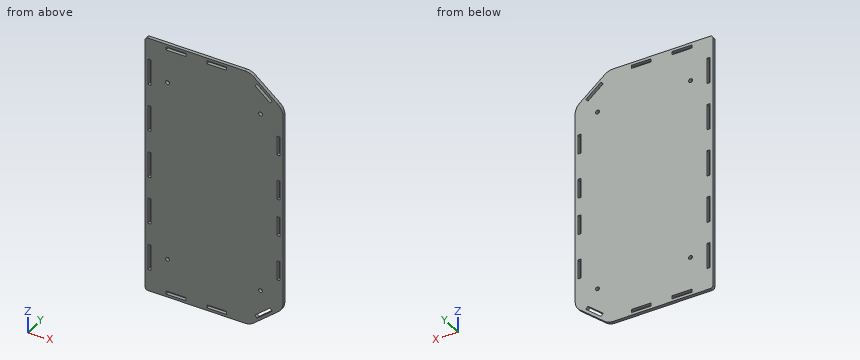
from build123d import *

# Parameters (mm, degrees)
SKETCH1_R           = 1.5
SKETCH1_W           = 15
SKETCH1_H           = 2.5
SKETCH1_W_2         = 2.5
SKETCH1_H_2         = 15
SKETCH1_H_3         = 20
BOSS_EXTRUDE1_DEPTH = 1.25
FILLET1_R           = 10
FILLET2_R           = 2


with BuildPart() as part:
    # Sketch1 → Boss-Extrude1 (new, symmetric)
    with BuildSketch(Plane(origin=(0, 0, 0), x_dir=(1, 0, 0), z_dir=(0, 1, 0))):
        Polygon((-52, -100), (27, -100), (52, -79.022509221), (52, 79.022509221), (27, 100), (-52, 100), align=None)
        with Locations(Location((35.127158073, -70, 0), (0, 0, 270))):
            Circle(SKETCH1_R, mode=Mode.SUBTRACT)
        with Locations(Location((35.127158073, 70, 0), (0, 0, 270))):
            Circle(SKETCH1_R, mode=Mode.SUBTRACT)
        with Locations(Location((-35.127158073, 70, 0), (0, 0, 270))):
            Circle(SKETCH1_R, mode=Mode.SUBTRACT)
        with Locations(Location((-35.127158073, -70, 0), (0, 0, 270))):
            Circle(SKETCH1_R, mode=Mode.SUBTRACT)
        with Locations((-28.71, -96.75)):
            Rectangle(SKETCH1_W, SKETCH1_H, mode=Mode.SUBTRACT)
        with Locations((2.08, -96.75)):
            Rectangle(SKETCH1_W, SKETCH1_H, mode=Mode.SUBTRACT)
        with Locations((-28.71, 96.75)):
            Rectangle(SKETCH1_W, SKETCH1_H, mode=Mode.SUBTRACT)
        with Locations((2.08, 96.75)):
            Rectangle(SKETCH1_W, SKETCH1_H, mode=Mode.SUBTRACT)
        Polygon((30.862122433, -90.884961689), (32.469091457, -92.800072797), (43.959758104, -83.158258651), (42.35278908, -81.243147544), align=None, mode=Mode.SUBTRACT)
        with Locations((48.75, 14.424124759)):
            Rectangle(SKETCH1_W_2, SKETCH1_H_2, mode=Mode.SUBTRACT)
        with Locations((48.75, -49.424124759)):
            Rectangle(SKETCH1_W_2, SKETCH1_H_2, mode=Mode.SUBTRACT)
        with Locations((48.75, -14.424124759)):
            Rectangle(SKETCH1_W_2, SKETCH1_H_2, mode=Mode.SUBTRACT)
        with Locations((48.75, 49.424124759)):
            Rectangle(SKETCH1_W_2, SKETCH1_H_2, mode=Mode.SUBTRACT)
        Polygon((42.35278908, 81.243147544), (30.862122433, 90.884961689), (32.469091457, 92.800072797), (43.959758104, 83.158258651), align=None, mode=Mode.SUBTRACT)
        with Locations((-48.75, -36.666666667)):
            Rectangle(SKETCH1_W_2, SKETCH1_H_3, mode=Mode.SUBTRACT)
        with Locations((-48.75, -73.333333333)):
            Rectangle(SKETCH1_W_2, SKETCH1_H_3, mode=Mode.SUBTRACT)
        with Locations((-48.75, 0)):
            Rectangle(SKETCH1_W_2, SKETCH1_H_3, mode=Mode.SUBTRACT)
        with Locations((-48.75, 36.666666667)):
            Rectangle(SKETCH1_W_2, SKETCH1_H_3, mode=Mode.SUBTRACT)
        with Locations((-48.75, 73.333333333)):
            Rectangle(SKETCH1_W_2, SKETCH1_H_3, mode=Mode.SUBTRACT)
    extrude(amount=BOSS_EXTRUDE1_DEPTH, both=True)

    # Fillet1
    fillet1_edges = [part.edges().sort_by_distance(p)[0] for p in [
        (27, 0, -100),
        (52, 0, -79.022509221),
        (52, 0, 79.022509221),
        (27, 0, 100),
    ]]
    fillet(fillet1_edges, radius=FILLET1_R)

    # Fillet2
    fillet2_edges = [part.edges().sort_by_distance(p)[0] for p in [
        (-52, 0, 100),
        (-52, 0, -100),
    ]]
    fillet(fillet2_edges, radius=FILLET2_R)


solid = part.part
Work out the finished part from the listing and answer in its coordinate system (mm). Round coordinates to 2 decimals unless told otherwise and drop trailing zeros. Write each loop counter-clockwise with the first axis right and the second up, starting at its lowest first coordinate (ties: lowest second). Pieces come first, ordered by that corner, then holes.
1) Given pin 1 Ø0.8 at (y, z) = (0.5, 96.5) entering from +X; pin 2 Ø0.8 at (x, y) = (48.5, 0) entering from +Z (3 decimals); pin 3 Ø1.2 at (y, z) = (-0.5, 97) entering from +X, each flat-ended and moving along its own axis, determine where each tip first touches the part or whether it passes through.
2) A cutting plane is placed at C-C (y = 0.4). Give the number of separate pieces and of enclosed holes in the cut face, plus the area to 3 significant figures.
3) A cutting plane is placed at A-A (x = -24). Give the vertices of the cut face in (y, z).
4) A cutting plane is placed at B-B (z = -3). Give the vertices of the cut face in (x, y), plus the area to 3 significant figures.
5) Straight lines are drawn through the part: line 1 (Z direction, x = 9.5, y = 1.1); line 2 (X direction, y = 0.75, z = 70); line 3 (X direction, y = -0.9, z = -8). For each, find the intervals that lie inside material, in ascending order.
Completed:
1. pin 1: stops at x = 31.65
1. pin 2: stops at z = 82.295
1. pin 3: stops at x = 31.29
2. separate pieces: 1
2. enclosed holes: 19
2. area: 19,600 mm2
3. outline: (-1.25, -100) - (1.25, -100) - (1.25, -98) - (-1.25, -98) - close; (-1.25, -95.5) - (1.25, -95.5) - (1.25, 95.5) - (-1.25, 95.5) - close; (-1.25, 98) - (1.25, 98) - (1.25, 100) - (-1.25, 100) - close
4. outline: (-52, -1.25) - (-50, -1.25) - (-50, 1.25) - (-52, 1.25) - close; (-47.5, -1.25) - (52, -1.25) - (52, 1.25) - (-47.5, 1.25) - close
4. area: 254 mm2
5. line 1: z = -100 to -98, -95.5 to 95.5, 98 to 100
5. line 2: x = -52 to -50, -47.5 to -36.63, -33.63 to 33.63, 36.63 to 52
5. line 3: x = -52 to -50, -47.5 to 47.5, 50 to 52
